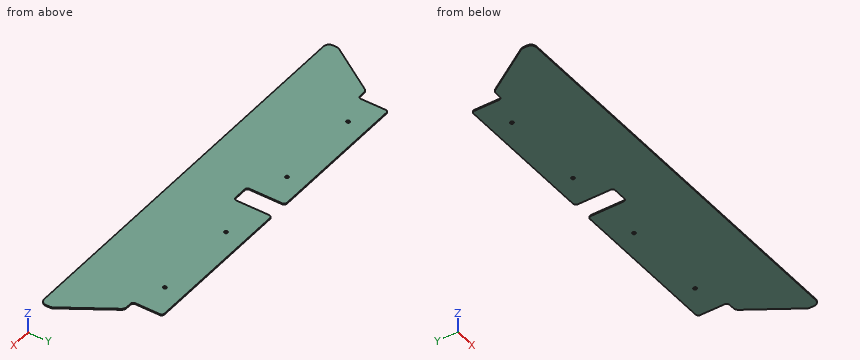
```python
from build123d import *

# Parameters (mm, degrees)
F1_DEPTH = 2


with BuildPart() as f1:
    # F0 (on Top) → F1 (new body)
    with BuildSketch(Plane.XY):
        with BuildLine():
            Line((265, 0), (5, 0))
            ThreePointArc((5, 0), (1.464466, -1.464466), (0, -5))
            Line((0, -5), (0, -50))
            ThreePointArc((0, -50), (-1.464466, -53.535534), (-5, -55))
            Line((-5, -55), (-14.575301, -55))
            ThreePointArc((-14.575301, -55), (-19.34359, -56.210039), (-22.957917, -59.547316))
            Line((-22.957917, -59.547316), (-78.382615, -144.753785))
            ThreePointArc((-78.382615, -144.753785), (-79.587131, -147.362717), (-80, -150.206469))
            Line((-80, -150.206469), (-80, -157.240251))
            ThreePointArc((-80, -157.240251), (-77.071068, -164.311319), (-70, -167.240251))
            Line((-70, -167.240251), (660, -167.240251))
            ThreePointArc((660, -167.240251), (667.071068, -164.311319), (670, -157.240251))
            Line((670, -157.240251), (670, -150.206469))
            ThreePointArc((670, -150.206469), (669.587131, -147.362717), (668.382615, -144.753785))
            Line((668.382615, -144.753785), (612.957917, -59.547316))
            ThreePointArc((612.957917, -59.547316), (609.34359, -56.210039), (604.575301, -55))
            Line((604.575301, -55), (595, -55))
            ThreePointArc((595, -55), (591.464466, -53.535534), (590, -50))
            Line((590, -50), (590, -5))
            ThreePointArc((590, -5), (588.535534, -1.464466), (585, 0))
            Line((585, 0), (309, 0))
            ThreePointArc((309, 0), (305.464466, -1.464466), (304, -5))
            Line((304, -5), (304, -35))
            Line((304, -35), (304, -55))
            Line((304, -55), (304, -65))
            ThreePointArc((304, -65), (302.535534, -68.535534), (299, -70))
            Line((299, -70), (275, -70))
            ThreePointArc((275, -70), (271.464466, -68.535534), (270, -65))
            Line((270, -65), (270, -55))
            Line((270, -55), (270, -35))
            Line((270, -35), (270, -5))
            ThreePointArc((270, -5), (268.535534, -1.464466), (265, 0))
        make_face()
        with BuildLine():
            ThreePointArc((52, -35), (55, -32), (58, -35))
            ThreePointArc((58, -35), (55, -38), (52, -35))
        make_face(mode=Mode.SUBTRACT)
        with BuildLine():
            ThreePointArc((212, -35), (215, -32), (218, -35))
            ThreePointArc((218, -35), (215, -38), (212, -35))
        make_face(mode=Mode.SUBTRACT)
        with BuildLine():
            ThreePointArc((377, -35), (374, -38), (371, -35))
            ThreePointArc((371, -35), (374, -32), (377, -35))
        make_face(mode=Mode.SUBTRACT)
        with BuildLine():
            ThreePointArc((537, -35), (534, -38), (531, -35))
            ThreePointArc((531, -35), (534, -32), (537, -35))
        make_face(mode=Mode.SUBTRACT)
    extrude(amount=F1_DEPTH)


solid = f1.part
```
The listing builds one solid part. Answer for the finished solid, in the listing's coordinates (mm). Give positions to 0.01 mm unless a question says otherwise; leave off trailing zeros. Order: outer loops, then holes, each group sorted by start corner. A loop starts at its lowest first (then second) coordinate and runs counter-clockwise, first axis right, second up. Notation, with made-up numbers: M 57,4.25 L 97,4.25 A21 ccw 97,26.25 Z; hole C 28.25,19.25 d3. An arc over 180 degrees is marked long. Put each result on its own line as item: value. Start each with the question number.
Item 1: The part is cut by section D-D, the plane y = -78. Determine the outline of the cut face in (x, z), and give its area (3 significant figures).
Item 2: The part is cut by section A-A, the plane y = -11.5. Determine the outline of the cut face in (x, z), and give its area (3 significant figures).
Item 3: The part is cut by section B-B, the plane z = 1.35. State how many separate pieces and enclosed holes the cut face has, and give its area (3 significant figures).
Item 4: Find the intervals of material crossed by line 1 along Y through (x, z) = (215, 0.95); line 2 along X through (y, z) = (-12.5, 0.3); line 3 along X through (y, z) = (-53, 1.2), in increasing order.
Item 5: Flat-ended cylindrical pins translate along their axes: P1, Ø1, axis at y = -130, z = 1, coming from the +X side; P2, Ø1, axis at y = -145.5, z = 1, coming from the +X side; P3, Ø1, axis at x = 600, z = 1.5, coming from the +Y side; P4, Ø4, axis at x = 231.5, y = -92, coming from the -Z side. Find the tip coordinate at first contact, or state that the pin passes through.
Item 6: The part is cut by section C-C, the plane y = -129.5. Determine the outline of the cut face in (x, z).
Answer key:
1. outline: M -34.96,0 L 624.96,0 L 624.96,2 L -34.96,2 Z
1. area: 1,320 mm²
2. outline: M 0,0 L 270,0 L 270,2 L 0,2 Z; M 304,0 L 590,0 L 590,2 L 304,2 Z
2. area: 1,110 mm²
3. separate pieces: 1
3. enclosed holes: 4
3. area: 109,000 mm²
4. line 1: y = -167.24 to -38, -32 to 0
4. line 2: x = 0 to 270, 304 to 590
4. line 3: x = -1 to 270, 304 to 591
5. P1: stops at x = 659.11
5. P2: stops at x = 669.07
5. P3: stops at y = -55
5. P4: stops at z = 0
6. outline: M -68.46,0 L 658.46,0 L 658.46,2 L -68.46,2 Z
